```python
from build123d import *

# Parameters (mm, degrees)
SWEEP_1_PROFILE_R        = 5.5
FILLET_1_R               = 1
CUT_EXTRUDE_1_DEPTH      = 54.023579723
CUT_EXTRUDE_1_DEPTH_BACK = 54.023579723
FILLET_2_R               = 0.5
CUT_EXTRUDE_2_DEPTH      = 54.023579723
CUT_EXTRUDE_2_DEPTH_BACK = 54.023579723
SKETCH_11_W              = 2
SKETCH_11_H              = 3.5
CUT_EXTRUDE_3_DEPTH      = 54.023579723
CUT_EXTRUDE_3_DEPTH_BACK = 54.023579723
CUT_EXTRUDE_4_DEPTH      = 54.023579723
CUT_EXTRUDE_4_DEPTH_BACK = 54.023579723
FILLET_3_R               = 0.5


with BuildPart() as part:
    # 扫描1: sweep along a path in 草图2
    with BuildLine(Plane.XY) as sweep_1_path:
        Line((-22, -25), (-22, 0))
        ThreePointArc((-22, 0), (0, 22), (22, 0))
        Line((22, 0), (22, -45))
    # 扫描1 profile (on start of the path) → 扫描1 (sweep)
    with BuildSketch(Plane(origin=(-22, -25, 0), x_dir=(1, 0, 0), z_dir=(0, 1, 0))):
        Circle(SWEEP_1_PROFILE_R)
    sweep(path=sweep_1_path.line)

    # 圆角1
    fillet_1_edges = [part.edges().sort_by_distance(p)[0] for p in [
        (-27.5, -25, 0),
    ]]
    fillet(fillet_1_edges, radius=FILLET_1_R)

    # 草图10 → 切除-拉伸1 (cut, two sides: drawn at the far end of the back side and taken through both)
    with BuildSketch(Plane.XY.offset(-CUT_EXTRUDE_1_DEPTH_BACK)):
        Polygon((-16.5, -22.5), (-21.39690683, -22.5), (-16.5, -16.664093693), align=None)
    extrude(amount=CUT_EXTRUDE_1_DEPTH + CUT_EXTRUDE_1_DEPTH_BACK, mode=Mode.SUBTRACT)

    # 圆角2
    fillet_2_edges = [part.edges().sort_by_distance(p)[0] for p in [
        (-21.39690683, -22.5, 0),
    ]]
    fillet(fillet_2_edges, radius=FILLET_2_R)

    # 草图11 → 切除-拉伸2 (cut, two sides: drawn at the far end of the back side and taken through both)
    with BuildSketch(Plane.XY.offset(-CUT_EXTRUDE_2_DEPTH_BACK)):
        with Locations((26.5, -41.25)):
            Rectangle(SKETCH_11_W, SKETCH_11_H)
        with Locations((17.5, -41.25)):
            Rectangle(SKETCH_11_W, SKETCH_11_H)
    extrude(amount=CUT_EXTRUDE_2_DEPTH + CUT_EXTRUDE_2_DEPTH_BACK, mode=Mode.SUBTRACT)

    # 草图12 → 切除-拉伸3 (cut, two sides: drawn at the far end of the back side and taken through both)
    with BuildSketch(Plane.XY.offset(-CUT_EXTRUDE_3_DEPTH_BACK)):
        Polygon((18.5, -39.5), (18.5, -28.5), (16.5, -27.345299462), (16.5, -39.5), align=None)
    extrude(amount=CUT_EXTRUDE_3_DEPTH + CUT_EXTRUDE_3_DEPTH_BACK, mode=Mode.SUBTRACT)

    # 草图13 → 切除-拉伸4 (cut, two sides: drawn at the far end of the back side and taken through both)
    with BuildSketch(Plane.XY.offset(-CUT_EXTRUDE_4_DEPTH_BACK)):
        Polygon((16.5, -22.5), (22, -22.5), (16.5, -15.945355241), align=None)
    extrude(amount=CUT_EXTRUDE_4_DEPTH + CUT_EXTRUDE_4_DEPTH_BACK, mode=Mode.SUBTRACT)

    # 圆角3
    fillet_3_edges = [part.edges().sort_by_distance(p)[0] for p in [
        (22, -22.5, 0),
    ]]
    fillet(fillet_3_edges, radius=FILLET_3_R)


solid = part.part
```
Could you check a few things on this model? Use its own coordinates, in mm. A direction names the side the tool comes from. Round coordinates to 2 decimals unless told otherwise and drop trailing zeros. Loops run counter-clockwise (first coordinate to the right, second up) from the corner with the lowest first, then second, coordinate; pieces in that order, holes last. Notation, with made-up numbers: (-13, 26.5) - (42, 26.5) arc R19 cw to (42, 58.5) - close; hole circle Ø5 at (48.25, 2). An arc over 180 degrees is marked (long way). Use CSV: the item, a comma, the result in double quotes.
Item 1: If we section it at B-B on y = -15: List the corners of the cut face in (x, z) for me.
Here are the results:
outline,"circle Ø11 at (-22, 0); circle Ø11 at (22, 0)"
Item 2: Will these pins go through, and if not, where does the flat tip stop? pin 1 (6 mm diameter, centred on y = 11, z = -2.5, fed in from +X); pin 2 (2.5 mm diameter, centred on y = -39, z = 1.5, fed in from -X); pin 3 (2 mm diameter, centred on x = 18, z = -1.5, fed in from +Y).
Here are the results:
pin 1,"stops at x = 26.09"
pin 2,"stops at x = 18.5"
pin 3,"stops at y = 21.41"
Item 3: If we mould it in two halves opening along X, with no side actions, what happens to faces 1 (the flat face through (18, -43, 0)), 2 (the flat face through (25.5, -41, 0)), 3 (the flat face through (19.474, -19.489, -0.076))? For each: pulls with the +X half, pulls with the -X half, needs draft (parallel to the pull), parting line crosses it, or undercut.
Here are the results:
face 1,"needs draft"
face 2,"pulls with the +X half"
face 3,"undercut"
Item 4: I need wall thicknesses on L1, parallel to X at y = -5.5, z = 2; L2, parallel to Y at x = 19.5, z = 3.5; L3, parallel to X at y = 11.5, z = -3.25. Which ranges of each line are inside material? Lowest first, please. Write a range as [from, to].
Here are the results:
L1,"x = [-27.12, -16.88], [16.88, 27.12]"
L2,"y = [-45, -22.5], [-19.52, 17.56]"
L3,"x = [-23.8, -13.27], [13.27, 23.8]"
Item 5: If we section it at C-C on y = -26: List the corners of the cut face in (x, z) for me, then the cut area to 3 significant figures.
Here are the results:
outline,"circle Ø11 at (22, 0)"
area,"95.0 mm²"
Item 6: For faces 4 (the flat face through (18.5, -36, 0)), 5 (the cylindrical face through (-27.495, -11.832, -0.242)), 6 (the flat face through (-19.1, -19.76, -0.07)), which set-ups out of +Z, -Z, +X, -X, +Y, -Y let a thin tool reach every point of the face, with its end or its side?
Here are the results:
face 4,"+Z, -Z, -X"
face 5,"-Y"
face 6,"+Z, -Z"
Item 7: If we section it at A-A on z = 0: List the corners of the cut face in (x, y) for me.
Here are the results:
outline,"(-27.5, -24) arc R1 ccw to (-26.5, -25) - (-17.5, -25) arc R1 ccw to (-16.5, -24) - (-16.5, -22.5) - (-20.32, -22.5) arc R0.5 cw to (-20.71, -21.68) - (-16.5, -16.66) - (-16.5, 0) arc R16.5 cw to (16.5, 0) - (16.5, -15.95) - (21.31, -21.68) arc R0.5 cw to (20.93, -22.5) - (16.5, -22.5) - (16.5, -27.35) - (18.5, -28.5) - (18.5, -43) - (16.5, -43) - (16.5, -45) - (27.5, -45) - (27.5, -43) - (25.5, -43) - (25.5, -39.5) - (27.5, -39.5) - (27.5, 0) arc R27.5 ccw to (-27.5, 0) - close"
